For this review, take the finished solid that the model builds, in its own axes (mm). Coordinates: 2 decimals unless noted, no trailing zeros. Write each loop counter-clockwise with the first axis right and the second up, starting at its lowest first coordinate (ties: lowest second). Pieces come first, ordered by that corner, then holes.
```python
from build123d import *

# Parameters (mm, degrees)
BOSS_EXTRUDE2_DEPTH      = 5.3975
SKETCH3_R                = 12.192
SKETCH3_R_2              = 12.1285
CUT_EXTRUDE2_DEPTH       = 6.3975
SKETCH5_W                = 19.05
SKETCH5_H                = 13.716
CUT_EXTRUDE3_DEPTH       = 40.64
SKETCH6_R                = 38.1
CUT_EXTRUDE4_DEPTH       = 6.3975
SKETCH11_R               = 1.651
CUT_EXTRUDE9_DEPTH       = 75.692
SKETCH13_R               = 1.651
CUT_EXTRUDE11_DEPTH      = 97.79
SKETCH15_R               = 3.175
CUT_EXTRUDE13_DEPTH      = 103.378
CUT_EXTRUDE13_DEPTH_BACK = 48.768


with BuildPart() as part:
    # Sketch1 → Boss-Extrude2 (new body)
    with BuildSketch(Plane.XY):
        with BuildLine():
            Line((-68.450525929, 30.48), (-55.750525929, 30.48))
            Line((-55.750525929, 30.48), (-55.750525929, -30.48))
            Line((-55.750525929, -30.48), (-68.450525929, -30.48))
            ThreePointArc((-68.450525929, -30.48), (0, -74.93), (68.450525929, -30.48))
            Line((68.450525929, -30.48), (55.750525929, -30.48))
            Line((55.750525929, -30.48), (55.750525929, 30.48))
            Line((55.750525929, 30.48), (68.450525929, 30.48))
            ThreePointArc((68.450525929, 30.48), (0, 74.93), (-68.450525929, 30.48))
        make_face()
    extrude(amount=BOSS_EXTRUDE2_DEPTH)

    # Sketch3 → Cut-Extrude2 (cut, through all)
    with BuildSketch(Plane(origin=(0, 0, 0), x_dir=(-1, 0, 0), z_dir=(0, 0, -1))):
        with Locations((-13.97, 0)):
            Circle(SKETCH3_R)
        with Locations((13.97, 0)):
            Circle(SKETCH3_R)
        with Locations((40.64, 0)):
            Circle(SKETCH3_R)
        with Locations((-43.105229381, -43.105229381)):
            Circle(SKETCH3_R_2)
        with Locations((14.224, -34.29)):
            Circle(SKETCH3_R_2)
        with Locations((14.224, 34.29)):
            Circle(SKETCH3_R_2)
        with Locations((-43.105229381, 43.105229381)):
            Circle(SKETCH3_R_2)
        with Locations((43.105229381, 43.105229381)):
            Circle(SKETCH3_R_2)
        with Locations((-14.224, 34.29)):
            Circle(SKETCH3_R_2)
        with Locations((-14.224, -34.29)):
            Circle(SKETCH3_R_2)
        with Locations((43.105229381, -43.105229381)):
            Circle(SKETCH3_R_2)
        with Locations((-40.64, 0)):
            Circle(SKETCH3_R)
    extrude(amount=-CUT_EXTRUDE2_DEPTH, mode=Mode.SUBTRACT)

    # Sketch5 → Cut-Extrude3 (cut)
    with BuildSketch(Plane(origin=(0, 0, 0), x_dir=(-1, 0, 0), z_dir=(0, 0, -1))):
        with Locations((0, 62.23)):
            Rectangle(SKETCH5_W, SKETCH5_H)
    extrude(amount=-CUT_EXTRUDE3_DEPTH, mode=Mode.SUBTRACT)

    # Sketch6 → Cut-Extrude4 (cut, through all)
    with BuildSketch(Plane.XY.offset(5.3975)):
        with Locations((0, -86.312058398)):
            Circle(SKETCH6_R)
    extrude(amount=-CUT_EXTRUDE4_DEPTH, mode=Mode.SUBTRACT)

    # Sketch11 → Cut-Extrude9 (cut)
    with BuildSketch(Plane(origin=(30.092005081, 4.08352975, -6.096), x_dir=(-1, 0, 0), z_dir=(0, 0, -1))):
        with Locations((63.757223581, 17.50647025)):
            Circle(SKETCH11_R)
        with Locations((63.757223581, -25.67352975)):
            Circle(SKETCH11_R)
        with Locations((-3.552776419, -25.67352975)):
            Circle(SKETCH11_R)
        with Locations((-3.552776419, 17.50647025)):
            Circle(SKETCH11_R)
    extrude(amount=-CUT_EXTRUDE9_DEPTH, mode=Mode.SUBTRACT)

    # Sketch13 → Cut-Extrude11 (cut)
    with BuildSketch(Plane(origin=(30.092005081, 4.08352975, -36.1315), x_dir=(-1, 0, 0), z_dir=(0, 0, -1))):
        with Locations((4.154396091, -49.728759131)):
            Circle(SKETCH13_R)
        with Locations((56.02961407, -49.728759131)):
            Circle(SKETCH13_R)
        with Locations((4.154396091, 41.38247025)):
            Circle(SKETCH13_R)
        with Locations((56.02961407, 41.38247025)):
            Circle(SKETCH13_R)
    extrude(amount=-CUT_EXTRUDE11_DEPTH, mode=Mode.SUBTRACT)

    # Sketch15 → Cut-Extrude13 (cut, two sides)
    with BuildSketch(Plane(origin=(30.092005081, 4.08352975, 0), x_dir=(-1, 0, 0), z_dir=(0, 0, -1))) as cut_extrude13_sk:
        with Locations((-16.897994919, 21.31647025)):
            Circle(SKETCH15_R)
        with Locations((77.082005081, 21.31647025)):
            Circle(SKETCH15_R)
        with Locations((30.092005081, 21.31647025)):
            Circle(SKETCH15_R)
        with Locations((77.082005081, -29.48352975)):
            Circle(SKETCH15_R)
        with Locations((30.092005081, -29.48352975)):
            Circle(SKETCH15_R)
        with Locations((-16.897994919, -29.48352975)):
            Circle(SKETCH15_R)
    extrude(amount=CUT_EXTRUDE13_DEPTH, mode=Mode.SUBTRACT)
    extrude(cut_extrude13_sk.sketch, amount=-CUT_EXTRUDE13_DEPTH_BACK, mode=Mode.SUBTRACT)


solid = part.part
```
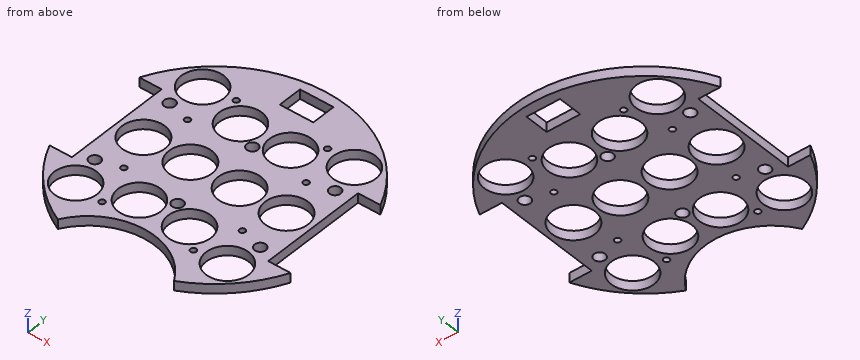
Q1. Add section C-C (y = -53.5). State the section outline as (x, z) points, then the cut area to 3 significant figures.
Ans:
outline: (-52.46, 0) - (-49.35, 0) - (-49.35, 5.4) - (-52.46, 5.4) - close; (-36.86, 0) - (-19.36, 0) - (-19.36, 5.4) - (-36.86, 5.4) - close; (19.36, 0) - (36.86, 0) - (36.86, 5.4) - (19.36, 5.4) - close; (49.35, 0) - (52.46, 0) - (52.46, 5.4) - (49.35, 5.4) - close
area: 222 mm2
Q2. Add section B-B (x = -46.99). State the section outline as (y, z) points (1 decimal), then the cut area to 3 significant figures.
Ans:
outline: (-58.4, 0) - (-54.6, 0) - (-54.6, 5.4) - (-58.4, 5.4) - close; (-31.6, 0) - (-28.6, 0) - (-28.6, 5.4) - (-31.6, 5.4) - close; (-22.2, 0) - (-10.4, 0) - (-10.4, 5.4) - (-22.2, 5.4) - close; (10.4, 0) - (22.2, 0) - (22.2, 5.4) - (10.4, 5.4) - close; (28.6, 0) - (31.6, 0) - (31.6, 5.4) - (28.6, 5.4) - close; (54.6, 0) - (58.4, 0) - (58.4, 5.4) - (54.6, 5.4) - close
area: 201 mm2
Q3. Clearance check with flat-ended pins moving along their axes: pin 1 Ø14.5 at (x, y) = (-13.97, 0) entering from -Z; pin 2 Ø1.6 at (x, z) = (-62.5, 2) entering from -Y; pin 3 Ø2 at (y, z) = (-41, 4.5) entering from -X; pin 4 Ø1.5 at (y, z) = (-16, 4) entering from -X. State where each tip first meets the part, or that it passes through.
Ans:
pin 1: passes through
pin 2: stops at y = -42.52
pin 3: stops at x = -63.36
pin 4: stops at x = -55.75
Q4. Add section A-A (y = -25.4). State the section outline as (x, z) points (1 decimal), then the cut area to 3 significant figures.
Ans:
outline: (-55.8, 0) - (-50.2, 0) - (-50.2, 5.4) - (-55.8, 5.4) - close; (-43.8, 0) - (-22.5, 0) - (-22.5, 5.4) - (-43.8, 5.4) - close; (-6, 0) - (-3.2, 0) - (-3.2, 5.4) - (-6, 5.4) - close; (3.2, 0) - (6, 0) - (6, 5.4) - (3.2, 5.4) - close; (22.5, 0) - (43.8, 0) - (43.8, 5.4) - (22.5, 5.4) - close; (50.2, 0) - (55.8, 0) - (55.8, 5.4) - (50.2, 5.4) - close
area: 321 mm2
Q5. Add section D-D (x = -13.97). State the section outline as (y, z) points, then the cut area to 3 significant figures.
Ans:
outline: (-50.87, 0) - (-46.42, 0) - (-46.42, 5.4) - (-50.87, 5.4) - close; (-22.16, 0) - (-12.19, 0) - (-12.19, 5.4) - (-22.16, 5.4) - close; (12.19, 0) - (22.16, 0) - (22.16, 5.4) - (12.19, 5.4) - close; (46.42, 0) - (73.62, 0) - (73.62, 5.4) - (46.42, 5.4) - close
area: 278 mm2
Q6. For probe 1 along Y at (x, z) = (0, 3.5) (3 decimals); probe 2 along Y at (x, z) = (48.5, 2.1); probe 3 along Y at (x, z) = (-36, 0.5), list the stretches that pass through material, from the lowest coordinate up.
Ans:
probe 1: y = -48.212 to -28.575, -22.225 to 22.225, 28.575 to 55.372, 69.088 to 74.93
probe 2: y = -57.12 to -53.97, -32.24 to -28.19, -22.61 to -9.32, 9.32 to 22.61, 28.19 to 32.24, 53.97 to 57.12
probe 3: y = -65.72 to -52.93, -33.28 to -11.27, 11.27 to 33.28, 52.93 to 65.72
